Design review of the part built by this model. Coordinates are the model's own, in mm. A direction names the side the tool comes from. Coordinates: 2 decimals unless noted, no trailing zeros. Order: outer loops, then holes, each group sorted by start corner. A loop starts at its lowest first (then second) coordinate and runs counter-clockwise, first axis right, second up. Notation, with made-up numbers: M 6.25,12.25 L 60.25,12.25 A18 cw 60.25,30.25 Z; hole C -29,33.5 d2. An arc over 180 degrees is marked long. Answer in a Markdown table with one row per item.
from build123d import *

# Parameters (mm, degrees)
BOX001_W     = 18
BOX001_H     = 2
BOX001_DEPTH = 10
BOX_W        = 20
BOX_H        = 40
BOX_DEPTH    = 10


with BuildPart() as sphere001:
    # Sphere001 → Sphere001 (revolve)
    with BuildSketch(Plane(origin=(4, 4, 10), x_dir=(1, 0, 0), z_dir=(0, -1, 0))):
        with BuildLine():
            ThreePointArc((0, -2), (2, 0), (0, 2))
            Line((0, 2), (0, -2))
        make_face()
    revolve(axis=Axis((4, 4, 10), (0, 0, 1)))


with BuildPart() as sphere002:
    # Sphere002 → Sphere002 (revolve)
    with BuildSketch(Plane(origin=(15, 4, 10), x_dir=(1, 0, 0), z_dir=(0, -1, 0))):
        with BuildLine():
            ThreePointArc((0, -2), (2, 0), (0, 2))
            Line((0, 2), (0, -2))
        make_face()
    revolve(axis=Axis((15, 4, 10), (0, 0, 1)))


with BuildPart() as sphere003:
    # Sphere003 → Sphere003 (revolve)
    with BuildSketch(Plane(origin=(4, 35, 10), x_dir=(1, 0, 0), z_dir=(0, -1, 0))):
        with BuildLine():
            ThreePointArc((0, -2), (2, 0), (0, 2))
            Line((0, 2), (0, -2))
        make_face()
    revolve(axis=Axis((4, 35, 10), (0, 0, 1)))


with BuildPart() as sphere004:
    # Sphere004 → Sphere004 (revolve)
    with BuildSketch(Plane(origin=(15, 15, 10), x_dir=(1, 0, 0), z_dir=(0, -1, 0))):
        with BuildLine():
            ThreePointArc((0, -2), (2, 0), (0, 2))
            Line((0, 2), (0, -2))
        make_face()
    revolve(axis=Axis((15, 15, 10), (0, 0, 1)))


with BuildPart() as sphere005:
    # Sphere005 → Sphere005 (revolve)
    with BuildSketch(Plane(origin=(10, 30.5, 10), x_dir=(1, 0, 0), z_dir=(0, -1, 0))):
        with BuildLine():
            ThreePointArc((0, -2), (2, 0), (0, 2))
            Line((0, 2), (0, -2))
        make_face()
    revolve(axis=Axis((10, 30.5, 10), (0, 0, 1)))


with BuildPart() as sphere006:
    # Sphere006 → Sphere006 (revolve)
    with BuildSketch(Plane(origin=(4, 15, 10), x_dir=(1, 0, 0), z_dir=(0, -1, 0))):
        with BuildLine():
            ThreePointArc((0, -2), (2, 0), (0, 2))
            Line((0, 2), (0, -2))
        make_face()
    revolve(axis=Axis((4, 15, 10), (0, 0, 1)))


with BuildPart() as sphere007:
    # Sphere007 → Sphere007 (revolve)
    with BuildSketch(Plane(origin=(15, 26, 10), x_dir=(1, 0, 0), z_dir=(0, -1, 0))):
        with BuildLine():
            ThreePointArc((0, -2), (2, 0), (0, 2))
            Line((0, 2), (0, -2))
        make_face()
    revolve(axis=Axis((15, 26, 10), (0, 0, 1)))


with BuildPart() as sphere:
    # Sphere → Sphere (revolve)
    with BuildSketch(Plane(origin=(10, 9.5, 10), x_dir=(1, 0, 0), z_dir=(0, -1, 0))):
        with BuildLine():
            ThreePointArc((0, -2), (2, 0), (0, 2))
            Line((0, 2), (0, -2))
        make_face()
    revolve(axis=Axis((10, 9.5, 10), (0, 0, 1)))


with BuildPart() as cube001:
    # Box001 → Box001 (new body)
    with BuildSketch(Plane(origin=(1, 19, 0), x_dir=(1, 0, 0), z_dir=(0, 0, 1))):
        with Locations((9, 1)):
            Rectangle(BOX001_W, BOX001_H)
    extrude(amount=BOX001_DEPTH)


with BuildPart() as cut008:
    # Box → Box (new body)
    with BuildSketch(Plane.XY):
        with Locations((10, 20)):
            Rectangle(BOX_W, BOX_H)
    extrude(amount=BOX_DEPTH)

    # Cut: cut Cube001
    add(cube001.part, mode=Mode.SUBTRACT)

    # Cut001: cut Sphere
    add(sphere.part, mode=Mode.SUBTRACT)

    # Cut002: cut Sphere007
    add(sphere007.part, mode=Mode.SUBTRACT)

    # Cut003: cut Sphere006
    add(sphere006.part, mode=Mode.SUBTRACT)

    # Cut004: cut Sphere005
    add(sphere005.part, mode=Mode.SUBTRACT)

    # Cut005: cut Sphere004
    add(sphere004.part, mode=Mode.SUBTRACT)

    # Cut006: cut Sphere003
    add(sphere003.part, mode=Mode.SUBTRACT)

    # Cut007: cut Sphere002
    add(sphere002.part, mode=Mode.SUBTRACT)

    # Cut008: cut Sphere001
    add(sphere001.part, mode=Mode.SUBTRACT)


solid = cut008.part
(1) Add section A-A, the plane z = 3.75. Give the boundary of the cut face in (x, y), and give its area (3 significant figures).
Return value:
| item | result |
|---|---|
| outline | M 0,0 L 20,0 L 20,40 L 0,40 Z; hole M 1,19 L 19,19 L 19,21 L 1,21 Z |
| area | 764 mm2 |
(2) Add section B-B, the plane x = 7. Give the boundary of the cut face in (y, z).
Return value:
| item | result |
|---|---|
| outline | M 0,0 L 19,0 L 19,10 L 0,10 Z; M 21,0 L 40,0 L 40,10 L 21,10 Z |
(3) Add section C-C, the plane x = 15.75. Give the boundary of the cut face in (y, z).
Return value:
| item | result |
|---|---|
| outline | M 0,0 L 19,0 L 19,10 L 16.85,10 A1.85 cw 13.15,10 L 5.85,10 A1.85 cw 2.15,10 L 0,10 Z; M 21,0 L 40,0 L 40,10 L 27.85,10 A1.85 cw 24.15,10 L 21,10 Z |
(4) For line 1 along Y through (x, z) = (9, 5.25); line 2 along Y through (x, z) = (13.75, 9); line 3 along X through (y, z) = (9, 9), list the stretches that pass through material, from the lowest coordinate up. Write a range as from..to.
Return value:
| item | result |
|---|---|
| line 1 | y = 0..19, 21..40 |
| line 2 | y = 0..2.8, 5.2..13.8, 16.2..19, 21..24.8, 27.2..40 |
| line 3 | x = 0..8.34, 11.66..20 |
(5) Insertion check: pin 1 Ø4 at (x, y) = (15.5, 21) entering from -Z. The pin has a flat end and moves straight along its axis. Give the tip position at first contact, or say it passes through.
Return value:
| item | result |
|---|---|
| pin 1 | stops at z = 0 |
(6) For faces 1 (the flat face through (1, 20, 5)), 2 (the flat face through (10, 40, 5)), list the 3-axis set-ups (+Z, -Z, +X, -X, +Y, -Y) from which the entire face can be reached by the end or side of a thin tool; tool diameter is ignored.
Return value:
| item | result |
|---|---|
| face 1 | +Z, -Z |
| face 2 | +Z, -Z, +X, -X, +Y |
(7) Add section D-D, the plane y = 13.5. Give the boundary of the cut face in (x, z).
Return value:
| item | result |
|---|---|
| outline | M 0,0 L 20,0 L 20,10 L 16.32,10 A1.32 cw 13.68,10 L 5.32,10 A1.32 cw 2.68,10 L 0,10 Z |
(8) Draft analysis for pull direction X (two halves, no side actions). For faces 3 (the flat face through (10, 0, 5)), 4 (the flat face through (20, 20, 5)), 5 (the flat face through (0, 20, 5)), 6 (the flat face through (10, 21, 5)), state which applies: pulls with the +X half, pulls with the -X half, needs draft (parallel to the pull), parting line crosses it, or undercut.
Return value:
| item | result |
|---|---|
| face 3 | needs draft |
| face 4 | pulls with the +X half |
| face 5 | pulls with the -X half |
| face 6 | undercut |
